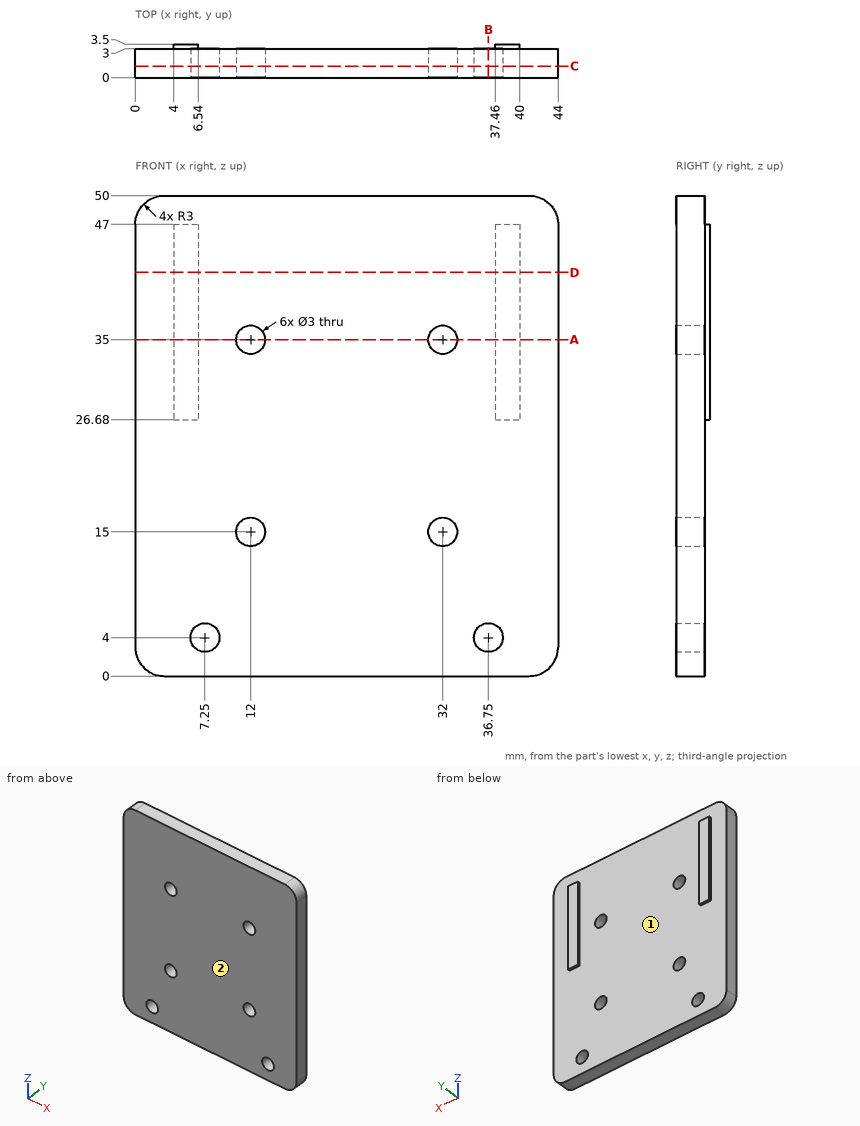
Input: dimensioned drawing with shaded views. Units: mm. Origin: part minimum x, y, z. Give positions to 0.01 mm unless a question says otherwise; leave off trailing zeros. Write each loop counter-clockwise with the first axis right and the second up, starting at its lowest first coordinate (ties: lowest second). Pieces come first, ordered by that corner, then holes.
1. Pin query (flat end, axial travel): P1, Ø4, axis at x = 36.75, z = 4, coming from the -Y side; P2, Ø13, axis at x = 16, z = 35.5, coming from the +Y side; P3, Ø2.5, axis at x = 7.25, z = 4, coming from the -Y side; P4, Ø0.6, axis at x = 5, y = 3.5, coming from the +Z side. Return the tip coordinate at first contact, or that it passes through.
2. Section query C-C, the plane y = 1.2. Return loops of the section in (x, z).
3. Draft query along X for the marked faces 1 and 2. Return one class per face: released by +X, released by -X, zero draft, split by the parting line, or undercut.
4. Section query D-D, the plane z = 42. Return loops of the section in (x, y).
5. Section query A-A, the plane z = 35. Return loops of the section in (x, y).
6. Line query: probe 1 along X at (y, z) = (0.95, 35); probe 2 along X at (y, z) = (2.4, 4); probe 3 along Z at (x, y) = (13, 1.1). Output: solid intervals per line, ascending.
7. Section query B-B, the plane x = 36.75. Return loops of the section in (y, z).
Computed:
1. P1: stops at y = 0
1. P2: stops at y = 3
1. P3: passes through
1. P4: stops at z = 47
2. outline: (0, 3) arc R3 ccw to (3, 0) - (41, 0) arc R3 ccw to (44, 3) - (44, 47) arc R3 ccw to (41, 50) - (3, 50) arc R3 ccw to (0, 47) - close; hole circle Ø3 at (7.25, 4); hole circle Ø3 at (12, 15); hole circle Ø3 at (12, 35); hole circle Ø3 at (32, 15); hole circle Ø3 at (32, 35); hole circle Ø3 at (36.75, 4)
3. face 1: undercut
3. face 2: zero draft
4. outline: (0, 0) - (44, 0) - (44, 3) - (40, 3) - (40, 3.5) - (37.46, 3.5) - (37.46, 3) - (6.54, 3) - (6.54, 3.5) - (4, 3.5) - (4, 3) - (0, 3) - close
5. outline: (0, 0) - (10.5, 0) - (10.5, 3) - (6.54, 3) - (6.54, 3.5) - (4, 3.5) - (4, 3) - (0, 3) - close; (13.5, 0) - (30.5, 0) - (30.5, 3) - (13.5, 3) - close; (33.5, 0) - (44, 0) - (44, 3) - (40, 3) - (40, 3.5) - (37.46, 3.5) - (37.46, 3) - (33.5, 3) - close
6. probe 1: x = 0 to 10.5, 13.5 to 30.5, 33.5 to 44
6. probe 2: x = 0 to 5.75, 8.75 to 35.25, 38.25 to 44
6. probe 3: z = 0 to 13.88, 16.12 to 33.88, 36.12 to 50
7. outline: (0, 0) - (3, 0) - (3, 2.5) - (0, 2.5) - close; (0, 5.5) - (3, 5.5) - (3, 50) - (0, 50) - close
